Geometry: final body of the model. Coordinates: model frame, mm. A direction names the side the tool comes from. Round coordinates to 2 decimals unless told otherwise and drop trailing zeros. Order: outer loops, then holes, each group sorted by start corner. A loop starts at its lowest first (then second) coordinate and runs counter-clockwise, first axis right, second up. Notation, with made-up numbers: M 10.5,37 L 50.5,37 A30 cw 50.5,66 Z; hole C 19,57 d9. An arc over 180 degrees is marked long. Put each result on its own line as item: value. Start each with the question number.
1) First-contact query: P1, Ø2.5, axis at x = 12, y = 6.5, coming from the -Z side; P2, Ø10, axis at x = 9, z = 5, coming from the -Y side. Flat tips, straight axial feed; report the tip coordinate or a pass-through.
2) Access query for faces 4 (the flat face through (0, 5, 0)), 5 (the cylindrical face through (4.35, 2.76, -19.3)), 6 (the flat face through (2, 6, 10)). Directions: +Z, -Z, +X, -X, +Y, -Y. A direction counts if a zero-diameter tool reaches every point of the face in a straight line with its end or side. Return the directions, or none.
3) Material intervals for probe 1 along Z at (x, y) = (0.5, 2.25); probe 2 along Y at (x, z) = (-5, -18.5); probe 3 along X at (y, z) = (5.85, -9.75), sorted ascending. Write a range as [from, to].
4) Section B-B, the plane z = -9.75. Return loops of the section in (x, y).
5) Draft query along Z for faces 1 (the flat face through (0, 8, -4)), 2 (the flat face through (-12, 4, -21.05)), 3 (the flat face through (0, 2, -14.25)). Return one class per face: pulls with the +Z half, pulls with the -Z half, needs draft (parallel to the pull), parting line crosses it, or undercut.
6) Section A-A, the plane x = -1. Return loops of the section in (y, z).
7) Section D-D, the plane x = 5. Return loops of the section in (y, z).
8) Section C-C, the plane y = 6.5. Return loops of the section in (x, z).
from build123d import *

# Parameters (mm, degrees)
SKETCH1_W                         = 36
SKETCH1_H                         = 33.5
SKETCH1_R                         = 1.4
SKETCH1_W_2                       = 3
SKETCH1_H_2                       = 21
SKETCH1_W_3                       = 16
SKETCH1_H_3                       = 3
BASE_DEPTH                        = 8
SKETCH3_W                         = 31
SKETCH3_H                         = 28.5
INTERIOR_CUTOUT_DEPTH             = 5
BASKET_MOUNTING_EDGE_DEPTH        = 8
SKETCH6_R                         = 1.4
BASKET_MOUNTING_SCREW_HOLES_DEPTH = 7
SKETCH7_W                         = 5
SKETCH7_H                         = 3
ZIP_TIE_HOLE_DEPTH                = 31.092565527
F_1MM_EDGE_FILLETS_R              = 1


with BuildPart() as part:
    # Sketch1 → Base (new body)
    with BuildSketch(Plane(origin=(0, 0, 0), x_dir=(1, 0, 0), z_dir=(0, 1, 0))):
        Rectangle(SKETCH1_W, SKETCH1_H)
        with Locations(Location((-11, -9.75, 0), (0, 0, 270))):
            Circle(SKETCH1_R, mode=Mode.SUBTRACT)
        with Locations(Location((-11, 9.75, 0), (0, 0, 270))):
            Circle(SKETCH1_R, mode=Mode.SUBTRACT)
        with Locations((12.5, 2.25)):
            Rectangle(SKETCH1_W_2, SKETCH1_H_2, mode=Mode.SUBTRACT)
        with Locations((2, -11.5)):
            Rectangle(SKETCH1_W_3, SKETCH1_H_3, mode=Mode.SUBTRACT)
    extrude(amount=BASE_DEPTH)

    # Sketch3 → Interior Cutout (cut)
    with BuildSketch(Plane.XZ):
        Rectangle(SKETCH3_W, SKETCH3_H)
    extrude(amount=-INTERIOR_CUTOUT_DEPTH, mode=Mode.SUBTRACT)

    # Sketch5 → Basket Mounting Edge (add)
    with BuildSketch(Plane(origin=(0, 0, 0), x_dir=(1, 0, 0), z_dir=(0, 1, 0))):
        with BuildLine():
            Line((-18, 16.75), (18, 16.75))
            Line((18, 16.75), (18, 22.75))
            Line((18, 22.75), (15.5, 22.75))
            ThreePointArc((15.5, 22.75), (15.002081528, 21.547918472), (13.8, 21.05))
            Line((13.8, 21.05), (11.2, 21.05))
            ThreePointArc((11.2, 21.05), (9.997918472, 21.547918472), (9.5, 22.75))
            Line((9.5, 22.75), (-9.5, 22.75))
            ThreePointArc((-9.5, 22.75), (-9.997918472, 21.547918472), (-11.2, 21.05))
            Line((-11.2, 21.05), (-13.8, 21.05))
            ThreePointArc((-13.8, 21.05), (-15.002081528, 21.547918472), (-15.5, 22.75))
            Line((-15.5, 22.75), (-18, 22.75))
            Line((-18, 22.75), (-18, 16.75))
        make_face()
    extrude(amount=BASKET_MOUNTING_EDGE_DEPTH)

    # Sketch6 → Basket Mounting Screw Holes (cut)
    with BuildSketch(Plane(origin=(0, 0, -22.75), x_dir=(-1, 0, 0), z_dir=(0, 0, -1))):
        with Locations((-5, 4)):
            Circle(SKETCH6_R)
        with Locations(Location((5, 4, 0), (0, 0, 180))):
            Circle(SKETCH6_R)
    extrude(amount=-BASKET_MOUNTING_SCREW_HOLES_DEPTH, mode=Mode.SUBTRACT)

    # Sketch7 → Zip Tie Hole (cut, through all)
    with BuildSketch(Plane(origin=(0, 8, 0), x_dir=(1, 0, 0), z_dir=(0, 1, 0))):
        with Locations((0, 18.75)):
            Rectangle(SKETCH7_W, SKETCH7_H)
    extrude(amount=-ZIP_TIE_HOLE_DEPTH, mode=Mode.SUBTRACT)

    # 1mm Edge Fillets
    f_1mm_edge_fillets_edges = [part.edges().sort_by_distance(p)[0] for p in [
        (18, 8, -3),
        (-18, 8, -3),
        (18, 4, 16.75),
        (-18, 4, 16.75),
        (0, 8, 16.75),
    ]]
    fillet(f_1mm_edge_fillets_edges, radius=F_1MM_EDGE_FILLETS_R)


solid = part.part
Result sheet:
1. P1: stops at z = -21.11
1. P2: stops at y = 5
2. face 4: -Y
2. face 5: -Z
2. face 6: +Y, -Y
3. probe 1: z = [-22.75, -20.25], [-17.25, -14.25], [14.25, 16.75]
3. probe 2: y = [0, 2.6], [5.4, 8]
3. probe 3: x = [-18, -12.4], [-9.6, 11], [14, 18]
4. outline: M -18,0 L -15.5,0 L -15.5,5 L -12.4,5 L -12.4,8 L -17,8 A1 ccw -18,7 Z; M -9.6,5 L 11,5 L 11,8 L -9.6,8 Z; M 14,5 L 15.5,5 L 15.5,0 L 18,0 L 18,7 A1 ccw 17,8 L 14,8 Z
5. face 1: needs draft
5. face 2: pulls with the -Z half
5. face 3: undercut
6. outline: M 0,-22.75 L 8,-22.75 L 8,-20.25 L 0,-20.25 Z; M 0,-17.25 L 8,-17.25 L 8,10 L 5,10 L 5,-14.25 L 0,-14.25 Z; M 0,14.25 L 5,14.25 L 5,13 L 8,13 L 8,15.75 A1 ccw 7,16.75 L 0,16.75 Z
7. outline: M 0,-22.75 L 2.6,-22.75 L 2.6,-15.75 L 5.4,-15.75 L 5.4,-22.75 L 8,-22.75 L 8,10 L 5,10 L 5,-14.25 L 0,-14.25 Z; M 0,14.25 L 5,14.25 L 5,13 L 8,13 L 8,15.75 A1 ccw 7,16.75 L 0,16.75 Z
8. outline: M -18,-22.75 L -15.5,-22.75 A1.7 cw -13.8,-21.05 L -11.2,-21.05 A1.7 cw -9.5,-22.75 L 9.5,-22.75 A1.7 cw 11.2,-21.05 L 13.8,-21.05 A1.7 cw 15.5,-22.75 L 18,-22.75 L 18,15.75 A1 ccw 17,16.75 L -17,16.75 A1 ccw -18,15.75 Z; hole C -11,-9.75 d2.8; hole C -11,9.75 d2.8; hole M -6,10 L 10,10 L 10,13 L -6,13 Z; hole M -2.5,-20.25 L 2.5,-20.25 L 2.5,-17.25 L -2.5,-17.25 Z; hole M 11,-12.75 L 14,-12.75 L 14,8.25 L 11,8.25 Z
